Part model, mm, in its own coordinate system. A direction names the side the tool comes from. Give positions to 0.01 mm unless a question says otherwise; leave off trailing zeros. Order: outer loops, then holes, each group sorted by start corner. A loop starts at its lowest first (then second) coordinate and runs counter-clockwise, first axis right, second up. Notation, with made-up numbers: (-27.5, -35.5) -> (17.5, -35.5) arc R22 ccw to (17.5, 2.5) -> close; hole circle Ø11 at (38.25, 44.5). An arc over 180 degrees is marked (long way). Write item = value, one per line. Start each with the question number.
(1) Saw through at A-A, the plane x = -76.2. List the corners of the cut face in (y, z) (3 decimals).
(2) Which spindle directions (+Z, -Z, +X, -X, +Y, -Y) get a long thin tool onto all of the face, cutting with end or side? Do faces 1 (the cylindrical face through (-64.086, 3.815, 1.61)), 2 (the flat face through (-61, 1, 3.175)). Say none if no direction does.
(3) Saw through at D-D, the plane z = 55.5. List the corners of the cut face in (x, y) (3 decimals), then the cut area to 3 significant figures.
(4) Saw through at B-B, the plane y = 0. List the corners of the cut face in (x, z) (3 decimals), then the cut area to 3 significant figures.
(5) Saw through at C-C, the plane y = 33.02. List the corners of the cut face in (x, z) (3 decimals).
(6) Probe line 1 along Y through (x, z) = (-76, 1); line 2 along Y through (x, z) = (-2.25, 101.6); line 3 along X through (y, z) = (4, 103) (3 decimals). List the from-to ranges inside material, lowest first. Write a range as from..to.
(7) Two-plate mould, pull along X, no slides. Class faces 3 (the cylindrical face through (-1.255, 1.067, 1.191)), 4 (the cylindrical face through (-78.288, -32.154, 1.61)), 5 (the flat face through (-63, 1, 0)): pulls with the +X half, pulls with the -X half, needs draft (parallel to the pull), parting line crosses it, or undercut.
(8) Flat gauge pins, fed straight in: pin 1 (5 mm diameter, centred on x = -115.5, y = -44, fed in from -Z); pin 2 (2.5 mm diameter, centred on x = -113.42, y = 0, fed in from +Z); pin 3 (2 mm diameter, centred on x = -56.5, y = 2, fed in from +Z) (3 decimals). Where does each tip first touch, or does it go through?
from build123d import *

# Parameters (mm, degrees)
BASE_FLANGE1_DEPTH = 76.2
SKETCH6_R          = 12.7
CUT_EXTRUDE1_DEPTH = 227.495696703
SKETCH7_R          = 2.2606
CUT_EXTRUDE2_DEPTH = 227.495696703
SKETCH9_R          = 2.286
CUT_EXTRUDE3_DEPTH = 227.495696703
SKETCH10_R         = 3.556
CUT_EXTRUDE4_DEPTH = 229.6


# Sheet-metal steps are written as plain solids
with BuildPart() as part:
    # Sketch1 → Base-Flange1 (new, symmetric)
    with BuildSketch(Plane(origin=(0, 0, 0), x_dir=(1, 0, 0), z_dir=(0, 1, 0))):
        with BuildLine():
            Line((-152.4, 0), (-4.175, 0))
            ThreePointArc((-4.175, 0), (-1.222829189, -1.222829189), (0, -4.175))
            Line((0, -4.175), (0, -152.4))
            Line((0, -152.4), (-3.175, -152.4))
            Line((-3.175, -152.4), (-3.175, -4.175))
            ThreePointArc((-3.175, -4.175), (-3.467893219, -3.467893219), (-4.175, -3.175))
            Line((-4.175, -3.175), (-152.4, -3.175))
            Line((-152.4, -3.175), (-152.4, 0))
        make_face()
    extrude(amount=BASE_FLANGE1_DEPTH, both=True)

    # Sketch6 → Cut-Extrude1 (cut, through all)
    with BuildSketch(Plane.XY.offset(3.175)):
        with Locations((-76.2, 0)):
            Circle(SKETCH6_R)
    extrude(amount=-CUT_EXTRUDE1_DEPTH, mode=Mode.SUBTRACT)

    # Sketch7 → Cut-Extrude2 (cut, through all)
    with BuildSketch(Plane.XY.offset(3.175)):
        with Locations((-76.2, 33.02)):
            Circle(SKETCH7_R)
        with Locations(Location((-76.2, -33.02, 0), (0, 0, 180))):
            Circle(SKETCH7_R)
    extrude(amount=-CUT_EXTRUDE2_DEPTH, mode=Mode.SUBTRACT)

    # Sketch9 → Cut-Extrude3 (cut, through all)
    with BuildSketch(Plane.XY.offset(3.175)):
        with Locations((-113.42361984, 0)):
            Circle(SKETCH9_R)
    extrude(amount=-CUT_EXTRUDE3_DEPTH, mode=Mode.SUBTRACT)

    # Sketch10 → Cut-Extrude4 (cut, through all)
    with BuildSketch(Plane(origin=(0, 0, 0), x_dir=(0, 0, -1), z_dir=(1, 0, 0))):
        with Locations((-54.975, 0)):
            Circle(SKETCH10_R)
        with Locations((-101.6, 0)):
            Circle(SKETCH10_R)
    extrude(amount=-CUT_EXTRUDE4_DEPTH, mode=Mode.SUBTRACT)


solid = part.part
Results list:
q1.outline = (-76.2, 0) -> (-35.281, 0) -> (-35.281, 3.175) -> (-76.2, 3.175) -> close; (-30.759, 0) -> (-12.7, 0) -> (-12.7, 3.175) -> (-30.759, 3.175) -> close; (12.7, 0) -> (30.759, 0) -> (30.759, 3.175) -> (12.7, 3.175) -> close; (35.281, 0) -> (76.2, 0) -> (76.2, 3.175) -> (35.281, 3.175) -> close
q2.face_1 = +Z, -Z
q2.face_2 = +Z, -X, +Y, -Y
q3.outline = (-3.175, -76.2) -> (0, -76.2) -> (0, -3.517) -> (-3.175, -3.517) -> close; (-3.175, 3.517) -> (0, 3.517) -> (0, 76.2) -> (-3.175, 76.2) -> close
q3.area = 462 mm^2
q4.outline = (-152.4, 0) -> (-115.71, 0) -> (-115.71, 3.175) -> (-152.4, 3.175) -> close; (-111.138, 0) -> (-88.9, 0) -> (-88.9, 3.175) -> (-111.138, 3.175) -> close; (-63.5, 0) -> (-4.175, 0) arc R4.175 ccw to (0, 4.175) -> (0, 51.419) -> (-3.175, 51.419) -> (-3.175, 4.175) arc R1 cw to (-4.175, 3.175) -> (-63.5, 3.175) -> close; (-3.175, 58.531) -> (0, 58.531) -> (0, 98.044) -> (-3.175, 98.044) -> close; (-3.175, 105.156) -> (0, 105.156) -> (0, 152.4) -> (-3.175, 152.4) -> close
q4.area = 814 mm^2
q5.outline = (-152.4, 0) -> (-78.461, 0) -> (-78.461, 3.175) -> (-152.4, 3.175) -> close; (-73.939, 0) -> (-4.175, 0) arc R4.175 ccw to (0, 4.175) -> (0, 152.4) -> (-3.175, 152.4) -> (-3.175, 4.175) arc R1 cw to (-4.175, 3.175) -> (-73.939, 3.175) -> close
q6.line_1 = -76.2..-35.27, -30.77..-12.7, 12.7..30.77, 35.27..76.2
q6.line_2 = -76.2..-3.56, 3.56..76.2
q6.line_3 = -3.175..0
q7.face_3 = pulls with the +X half
q7.face_4 = undercut
q7.face_5 = needs draft
q8.pin_1 = 0
q8.pin_2 = through
q8.pin_3 = 3.175
